Part model, mm, in its own coordinate system. A direction names the side the tool comes from. Round coordinates to 2 decimals unless told otherwise and drop trailing zeros. Order: outer loops, then holes, each group sorted by start corner. A loop starts at its lowest first (then second) coordinate and runs counter-clockwise, first axis right, second up. Notation, with made-up numbers: (0.25, 55) - (55.25, 55) arc R14 cw to (55.25, 62) - close; hole circle Ø3 at (41, -3.5). An arc over 180 degrees is marked (long way). Return JSON: item names as keys, results as strings. Group by question number.
Item 1: Tool access for faces 1 (the face through (3, 0, -5.013)), 2 (the face through (0, 5, -2)), 3 (the face through (56.86, -1.802, 5.723)): list every direction of +Z, -Z, +X, -X, +Y, -Y with a clear straight run to the whole face (end or side of a thin tool).
Item 2: Probe probe 1 along X at (y, z) = (6.75, 0.5); probe 2 along Y at (x, z) = (41.5, -3.75); probe 3 along Z at (x, y) = (9, 2.5). List the from-to ranges inside material, lowest first.
Item 3: Drop flat-ended pins along their axis: pin 1 (1.2 mm diameter, centred on y = 5, z = -0.5, fed in from -X); pin 2 (0.8 mm diameter, centred on y = 2.5, z = 4, fed in from -X); pin 3 (1 mm diameter, centred on x = 82, y = 4.5, fed in from +Z); pin 4 (8 mm diameter, centred on x = 40, z = 6, fed in from -Y). Give the stop position or say it passes through.
Item 4: Saw through at A-A on x = 54. List the corners of the cut face in (y, z).
```python
from build123d import *

# Parameters (mm, degrees)
FILLET1_R       = 0.6
FILLET2_R       = 1.2
HEX_2_DEPTH     = 6
THDSCHPAT_COUNT = 21
THDSCHPAT_PITCH = 1.714285714


with BuildPart() as part:
    # BodySke → Base-Revolve (revolve)
    with BuildSketch(Plane.XY, mode=Mode.PRIVATE) as base_revolve_sk:
        Polygon((0, 0), (0, 9), (12, 9), (12, 6), (91.036, 6), (92, 5.036), (92, 0), align=None)
    revolve(base_revolve_sk.sketch.rotate(Axis((-31.75, 0, 0), (1, 0, 0)), 90), axis=Axis((-31.75, 0, 0), (1, 0, 0)))  # turned: the seam where the file's is

    # Fillet1
    fillet1_edges = [part.edges().sort_by_distance(p)[0] for p in [
        (12, 0, -6),
    ]]
    fillet(fillet1_edges, radius=FILLET1_R)

    # Fillet2
    fillet2_edges = [part.edges().sort_by_distance(p)[0] for p in [
        (0, 0, -9),
    ]]
    fillet(fillet2_edges, radius=FILLET2_R)

    # Sketch2 → Hex-PreBroach (revolve, cut)
    with BuildSketch(Plane.XY, mode=Mode.PRIVATE) as hex_prebroach_sk:
        Polygon((0, 5.0125), (6, 5.0125), (8.893968224, 0), (0, 0), align=None)
    revolve(hex_prebroach_sk.sketch.rotate(Axis((0, 0, 0), (1, 0, 0)), 90), axis=Axis((0, 0, 0), (1, 0, 0)), mode=Mode.SUBTRACT)  # turned: the seam where the file's is

    # Sketch3 → Hex 2 (cut)
    with BuildSketch(Plane(origin=(0, 0, 0), x_dir=(0, 0.5, 0.866025404), z_dir=(-1, 0, 0))):
        Polygon((2.893968224, 5.0125), (-2.893968224, 5.0125), (-5.787936449, 0), (-2.893968224, -5.0125), (2.893968224, -5.0125), (5.787936449, 0), align=None)
    extrude(amount=-HEX_2_DEPTH, mode=Mode.SUBTRACT)

    # ThdSchSke → ThreadSchematic (revolve, cut)
    with BuildSketch(Plane.XY, mode=Mode.PRIVATE) as threadschematic_sk:
        Polygon((56, -5.036), (55.324999933, -6), (55.324999933, -7.5), (56.675000067, -7.5), (56.675000067, -6), align=None)
    threadschematic = revolve(threadschematic_sk.sketch.rotate(Axis((-3.175, 0, 0), (1, 0, 0)), 270), axis=Axis((-3.175, 0, 0), (1, 0, 0)), mode=Mode.SUBTRACT)  # turned: the seam where the file's is

    # ThdSchPat: ThreadSchematic ×21
    with Locations(*[(i * THDSCHPAT_PITCH, 0, 0) for i in range(1, THDSCHPAT_COUNT)]):
        add(threadschematic, mode=Mode.SUBTRACT)


solid = part.part
```
Filled in:
{
 "1": {"face 1": "-X", "face 2": "+Z, -Z, -X, +Y, -Y", "face 3": "+X"},
 "2": {"probe 1": "x = 0 to 12", "probe 2": "y = -4.68 to 4.68", "probe 3": "z = -8.65 to 8.65"},
 "3": {"pin 1": "stops at x = 0", "pin 2": "stops at x = 6", "pin 3": "stops at z = 4.3", "pin 4": "stops at y = -5.66"},
 "4": {"outline": "circle Ø12 at (0, 0)"}
}
